from build123d import *

# Parameters (mm, degrees)
BOSS_EXTRUDE1_DEPTH = 2
SKETCH3_R           = 3.2512
BOSS_EXTRUDE2_DEPTH = 5


with BuildPart() as part:
    # Sketch2 → Boss-Extrude1 (new body)
    with BuildSketch(Plane.XY):
        Polygon((16.575197596, -19.009332943), (-16.575197596, -19.009332943), (-19.089797596, -16.494732943), (-19.089797596, 16.494732943), (-16.575197596, 19.009332943), (16.575197596, 19.009332943), (19.089797596, 16.494732943), (19.089797596, -16.494732943), align=None)
    extrude(amount=BOSS_EXTRUDE1_DEPTH)

    # Sketch3 → Boss-Extrude2 (add)
    with BuildSketch(Plane.XY.offset(2)):
        Circle(SKETCH3_R)
    extrude(amount=BOSS_EXTRUDE2_DEPTH)


solid = part.part
Geometry: final body of the model. Coordinates: model frame, mm. A direction names the side the tool comes from. Give positions to 0.01 mm unless a question says otherwise; leave off trailing zeros. Loops run counter-clockwise (first coordinate to the right, second up) from the corner with the lowest first, then second, coordinate; pieces in that order, holes last. Notation, with made-up numbers: (-37, 9) -> (-31, 9) arc R32 cw to (-31, 36) -> close; hole circle Ø6 at (-16.75, 80.5). An arc over 180 degrees is marked (long way). Put each result on its own line as item: value.
1. Cut plane C-C (z = 3.5). Return the cut outline in (x, y).
Taken from the geometry:
outline: circle Ø6.5 at (0, 0)
2. Cut plane D-D (x = -13). Return the cut outline in (y, z), plus the area to 3 significant figures.
Taken from the geometry:
outline: (-19.01, 0) -> (19.01, 0) -> (19.01, 2) -> (-19.01, 2) -> close
area: 76.0 mm2
3. Set-up query: faces 1 (the flat face through (-19.09, 0, 1)), 2 (the cylindrical face through (-0.423, 3.224, 4.465)). Return all of +Z, -Z, +X, -X, +Y, -Y with unobstructed straight access to the full face (end or side cutting, diameter ignored); none if empty.
Taken from the geometry:
face 1: +Z, -Z, -X, +Y, -Y
face 2: +Z
4. Pin query (flat end, axial travel): P1, Ø6, axis at x = -14.5, y = -1.5, coming from the +Z side. Return the tip coordinate at first contact, or that it passes through.
Taken from the geometry:
P1: stops at z = 2
5. Ray query, line 1 along Z through (x, y) = (15, -8); line 2 along Y through (x, z) = (0.5, 5.5); line 3 along X through (y, z) = (-17, 1). Return the intervals inside material, ascending. Write a range as [from, to].
Taken from the geometry:
line 1: z = [0, 2]
line 2: y = [-3.21, 3.21]
line 3: x = [-18.58, 18.58]
6. Cut plane A-A (y = 0). Return the cut outline in (x, z).
Taken from the geometry:
outline: (-19.09, 0) -> (19.09, 0) -> (19.09, 2) -> (3.25, 2) -> (3.25, 7) -> (-3.25, 7) -> (-3.25, 2) -> (-19.09, 2) -> close
7. Cut plane B-B (x = 0). Return the cut outline in (y, z).
Taken from the geometry:
outline: (-19.01, 0) -> (19.01, 0) -> (19.01, 2) -> (3.25, 2) -> (3.25, 7) -> (-3.25, 7) -> (-3.25, 2) -> (-19.01, 2) -> close
